Geometry: final body of the model. Coordinates: model frame, mm. Face numbers are marked on the shaded views. A direction names the side the tool comes from. Give positions to 0.01 mm unless a question says otherwise; leave off trailing zeros. Loops run counter-clockwise (first coordinate to the right, second up) from the corner with the lowest first, then second, coordinate; pieces in that order, holes last. Notation, with made-up numbers: (79, 60.5) -> (113, 60.5) arc R26 cw to (113, 94.5) -> close; hole circle Ø3 at (72.5, 44.25). An arc over 180 degrees is marked (long way). One line per item, written item: value. Start each with the question number.
from build123d import *

# Parameters (mm, degrees)
SKETCH1_R           = 10
SKETCH1_R_2         = 7.5
SKETCH4_W           = 30
SKETCH4_H           = 30
SKETCH4_R           = 2.5
SKETCH4_R_2         = 7.5
BOSS_EXTRUDE3_DEPTH = 5


with BuildPart() as part:
    # Sweep3: sweep along a path in Sketch2
    with BuildLine(Plane.XY) as sweep3_path:
        ThreePointArc((0, 0), (-1.281289086, 35.324459387), (21.11820567, 62.668960981))
    # Sketch1 → Sweep3 (sweep)
    with BuildSketch(Plane(origin=(0, 0, 0), x_dir=(1, 0, 0), z_dir=(0, 1, 0))):
        Circle(SKETCH1_R)
        Circle(SKETCH1_R_2, mode=Mode.SUBTRACT)
    sweep(path=sweep3_path.line)

    # Sketch4 → Boss-Extrude3 (add)
    with BuildSketch(Plane(origin=(28.578554789, 3.610056753, 0), x_dir=(0, 0, -1), z_dir=(0.992115799, 0.125324544, 0))):
        with Locations((0, 59.528236809)):
            Rectangle(SKETCH4_W, SKETCH4_H)
        with Locations((-12, 71.528236809)):
            Circle(SKETCH4_R, mode=Mode.SUBTRACT)
        with Locations((12, 71.528236809)):
            Circle(SKETCH4_R, mode=Mode.SUBTRACT)
        with Locations((10, 48.035708089)):
            Circle(SKETCH4_R, mode=Mode.SUBTRACT)
        with Locations((-12, 48.035708089)):
            Circle(SKETCH4_R, mode=Mode.SUBTRACT)
        with Locations((0, 59.528236809)):
            Circle(SKETCH4_R_2, mode=Mode.SUBTRACT)
    extrude(amount=BOSS_EXTRUDE3_DEPTH)


solid = part.part
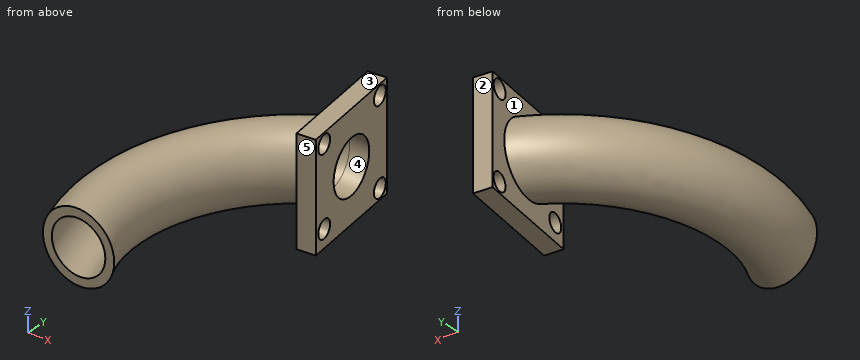
Item 1: Pin query (flat end, axial travel): pin 1 (10 mm diameter, centred on x = -1.5, z = 4, fed in from +Y); pin 2 (1.5 mm diameter, centred on x = 4.5, y = 17.5, fed in from +Z); pin 3 (3 mm diameter, centred on y = 39.5, z = -10.5, fed in from +X). Return the tip coordinate at first contact, or that it passes through.
Item 2: Section B-B, the plane x = 9. State how many separate pieces and enclosed holes the cut face has, then the cut area to 3 significant figures.
Item 3: Access query for the marked faces 1 and 2. Directions: +Z, -Z, +X, -X, +Y, -Y. A direction counts if a zero-diameter tool reaches every point of the face in a straight line with its end or side. Return the directions, or none.
Item 4: Mould query, pull axis X, two halves, no side actions, for the marked faces 3, 4 and 5. Classes: pulls with the +X half, pulls with the -X half, needs draft (parallel to the pull), parting line crosses it, or undercut.
Item 5: Section A-A, the plane z = 12.5. Output: boundary loops of the cut face in (x, y).
Item 6: Ray query, line 1 along X through (y, z) = (16.5, -0.25); line 2 along Z through (x, y) = (-9.5, 27.5); line 3 along Z through (x, y) = (-0.5, 30.5). Return the intervals inside material, ascending. Write a range as [from, to].
Geometry check:
1. pin 1: stops at y = 60
1. pin 2: stops at z = 5.45
1. pin 3: stops at x = 4.82
2. separate pieces: 2
2. enclosed holes: 1
2. area: 212 mm2
3. face 1: none
3. face 2: +Z, -Z, -X, +Y
4. face 3: needs draft
4. face 4: undercut
4. face 5: pulls with the +X half
5. outline: (19.24, 77.55) -> (19.31, 77) -> (24.27, 77.63) -> (24.2, 78.18) -> close; (19.92, 72.14) -> (22.25, 53.7) -> (27.21, 54.32) -> (24.88, 72.77) -> close; (22.87, 48.84) -> (23, 47.79) -> (27.96, 48.41) -> (27.83, 49.46) -> close
6. line 1: x = [-13.17, -10.81], [3.01, 5.23]
6. line 2: z = [-7.47, -3.46], [3.46, 7.47]
6. line 3: z = [-9.74, -7.15], [7.15, 9.74]
